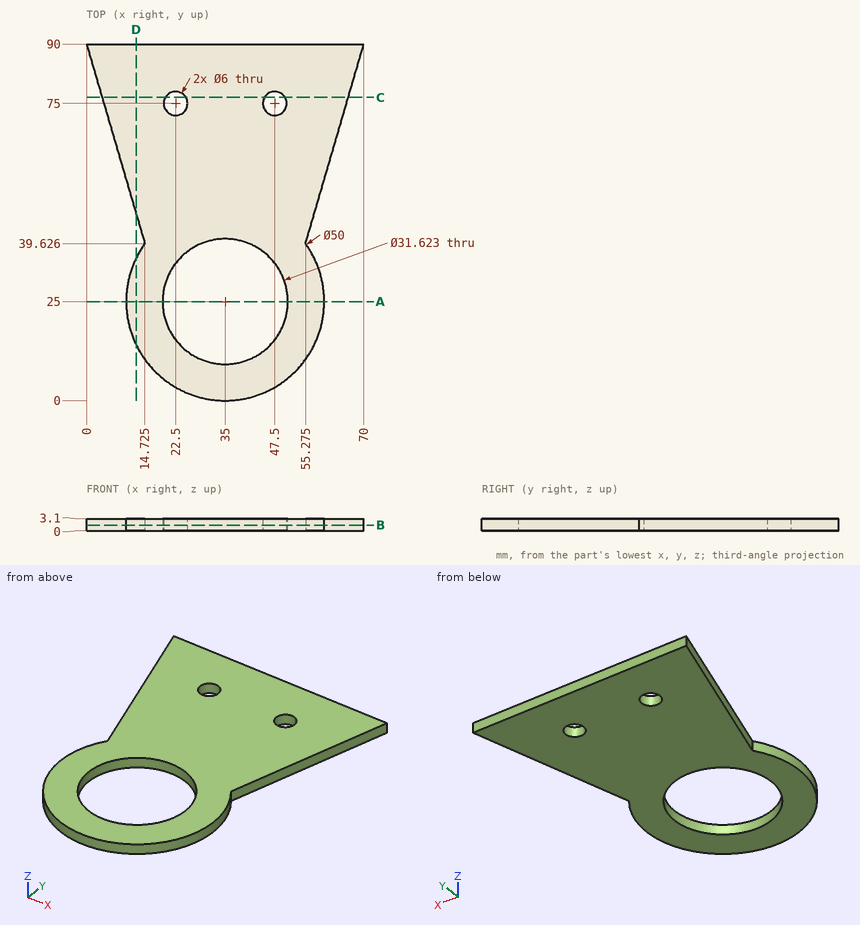
Answer from the drawing. Dimensions are ordinates in mm from the lowest x, y and z of the part. Give positions to 0.01 mm unless a question says otherwise; leave off trailing zeros. Loops run counter-clockwise (first coordinate to the right, second up) from the corner with the lowest first, then second, coordinate; pieces in that order, holes last. Notation, with made-up numbers: (70.5, 81.25) - (79.5, 81.25) arc R22 cw to (79.5, 103.25) - close; hole circle Ø4 at (36, 78). An arc over 180 degrees is marked (long way). Answer as a JSON object with one key per item and string values.
1. A cutting plane is placed at A-A (y = 25). Write down the section's boundary in (x, z).
Determined:
{"outline": "(10, 0) - (19.19, 0) - (19.19, 3.1) - (10, 3.1) - close; (50.81, 0) - (60, 0) - (60, 3.1) - (50.81, 3.1) - close"}
2. A cutting plane is placed at B-B (z = 1.45). Write down the section's boundary in (x, y) (1 decimal).
Determined:
{"outline": "(0, 90) - (14.7, 39.6) arc R25 ccw (long way) to (55.3, 39.6) - (70, 90) - close; hole circle Ø31.6 at (35, 25); hole circle Ø6 at (22.5, 75); hole circle Ø6 at (47.5, 75)"}
3. Find the intervals of material crossed by L1, parallel to Y at x = 35, z = 2; L2, parallel to Y at x = 22.5, z = 1.9; L3, parallel to X at y = 74, z = 1.1, in increasing order. Write a range as [from, to].
Determined:
{"L1": "[0, 9.19], [40.81, 90]", "L2": "[3.35, 15.32], [34.68, 72], [78, 90]", "L3": "[4.68, 19.67], [25.33, 44.67], [50.33, 65.32]"}
4. A cutting plane is placed at C-C (y = 76.5). Write down the section's boundary in (x, z).
Determined:
{"outline": "(3.95, 0) - (19.9, 0) - (19.9, 3.1) - (3.95, 3.1) - close; (25.1, 0) - (44.9, 0) - (44.9, 3.1) - (25.1, 3.1) - close; (50.1, 0) - (66.05, 0) - (66.05, 3.1) - (50.1, 3.1) - close"}
5. A cutting plane is placed at D-D (x = 12.5). Write down the section's boundary in (y, z), then the cut area to 3 significant figures.
Determined:
{"outline": "(14.1, 0) - (35.9, 0) - (35.9, 3.1) - (14.1, 3.1) - close; (47.24, 0) - (90, 0) - (90, 3.1) - (47.24, 3.1) - close", "area": "200 mm²"}
